from build123d import *

# Parameters (mm, degrees)
SKETCH_1_R      = 3.45
EXTRUDE_1_DEPTH = 0.3


with BuildPart() as part:
    # 草图1 → 凸台-拉伸1 (new body)
    with BuildSketch(Plane(origin=(0, 0, 0), x_dir=(1, 0, 0), z_dir=(0, 1, 0))):
        with BuildLine():
            Line((3.519943181, 1.9), (10, 1.9))
            ThreePointArc((10, 1.9), (11.9, 0), (10, -1.9))
            Line((10, -1.9), (3.519943181, -1.9))
            ThreePointArc((3.519943181, -1.9), (-4, 0), (3.519943181, 1.9))
        make_face()
        with Locations(Location((0, 0, 0), (0, 0, 270))):
            Circle(SKETCH_1_R, mode=Mode.SUBTRACT)
        with BuildLine():
            Line((10, -0.6), (8.5, -0.6))
            ThreePointArc((8.5, -0.6), (7.9, 0), (8.5, 0.6))
            Line((8.5, 0.6), (10, 0.6))
            ThreePointArc((10, 0.6), (10.6, 0), (10, -0.6))
        make_face(mode=Mode.SUBTRACT)
    extrude(amount=EXTRUDE_1_DEPTH)


solid = part.part
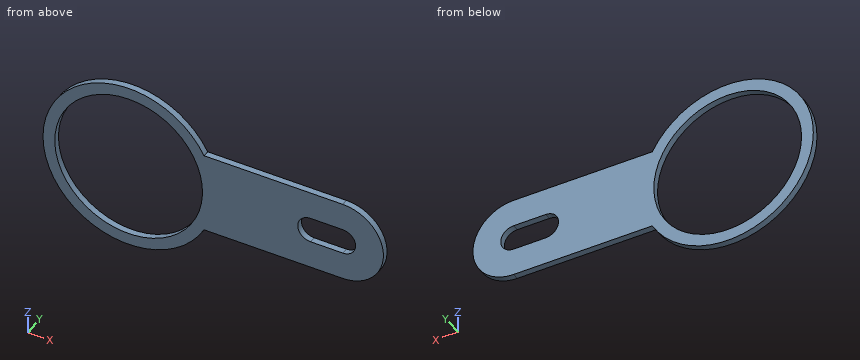
The listing builds one solid part. Answer for the finished solid, in the listing's coordinates (mm). Coordinates: 2 decimals unless noted, no trailing zeros. Loops run counter-clockwise (first coordinate to the right, second up) from the corner with the lowest first, then second, coordinate; pieces in that order, holes last. Notation, with made-up numbers: (39, 67) -> (63, 67) arc R35 cw to (63, 100) -> close; hole circle Ø11 at (4.5, 52). An arc over 180 degrees is marked (long way). Write item = value, one per line. Start each with the question number.
1) A cutting plane is placed at C-C (x = 0). Give the vertices of the cut face in (y, z), then the cut area to 3 significant figures.
2) A cutting plane is placed at A-A (z = 0). Give the vertices of the cut face in (x, y).
3) A cutting plane is placed at B-B (y = 0.15). Give the vertices of the cut face in (x, z), then the cut area to 3 significant figures.
4) A cutting plane is placed at D-D (z = 2.75). Give the vertices of the cut face in (x, y), then the cut area to 3 significant figures.
5) Straight lines are drawn through the part: line 1 (X direction, y = 0.15, z = 0); line 2 (X direction, y = 0.1, z = -0.25); line 3 (X direction, y = 0.1, z = -2.5). For each, find the intervals that lie inside material, in ascending order. Write a range as from..to.
Responses:
q1.outline = (0, -4) -> (0.3, -4) -> (0.3, -3.45) -> (0, -3.45) -> close; (0, 3.45) -> (0.3, 3.45) -> (0.3, 4) -> (0, 4) -> close
q1.area = 0.330 mm²
q2.outline = (-4, 0) -> (-3.45, 0) -> (-3.45, 0.3) -> (-4, 0.3) -> close; (3.45, 0) -> (7.9, 0) -> (7.9, 0.3) -> (3.45, 0.3) -> close; (10.6, 0) -> (11.9, 0) -> (11.9, 0.3) -> (10.6, 0.3) -> close
q3.outline = (3.52, -1.9) -> (10, -1.9) arc R1.9 ccw to (10, 1.9) -> (3.52, 1.9) arc R4 ccw (long way) to start; hole circle Ø6.9 at (0, 0); hole (8.5, -0.6) -> (10, -0.6) arc R0.6 ccw to (10, 0.6) -> (8.5, 0.6) arc R0.6 ccw to start
q3.area = 39.0 mm²
q4.outline = (-2.9, 0) -> (-2.08, 0) -> (-2.08, 0.3) -> (-2.9, 0.3) -> close; (2.08, 0) -> (2.9, 0) -> (2.9, 0.3) -> (2.08, 0.3) -> close
q4.area = 0.493 mm²
q5.line_1 = -4..-3.45, 3.45..7.9, 10.6..11.9
q5.line_2 = -3.99..-3.44, 3.44..7.95, 10.55..11.88
q5.line_3 = -3.12..-2.38, 2.38..3.12
